from build123d import *

# Parameters (mm, degrees)
SKETCH1_W           = 35
SKETCH1_H           = 35
BOSS_EXTRUDE1_DEPTH = 32
SKETCH2_R           = 16
SKETCH2_R_2         = 10.1
BOSS_EXTRUDE2_DEPTH = 10
SKETCH3_R           = 10
CUT_EXTRUDE1_DEPTH  = 25
SKETCH4_R           = 2
CUT_EXTRUDE2_DEPTH  = 20
SKETCH5_R           = 2
CUT_EXTRUDE3_DEPTH  = 20
SKETCH6_W           = 25
SKETCH6_H           = 25
SKETCH6_W_2         = 20.1
SKETCH6_H_2         = 20.1
BOSS_EXTRUDE3_DEPTH = 25
SKETCH7_R           = 2.5
CUT_EXTRUDE4_DEPTH  = 60.956234102
SKETCH8_R           = 2.5
CUT_EXTRUDE5_DEPTH  = 25
FILLET1_R           = 2
FILLET2_R           = 2
FILLET3_R           = 1
CHAMFER1_SIZE       = 2


with BuildPart() as part:
    # Sketch1 → Boss-Extrude1 (new body)
    with BuildSketch(Plane.XY):
        Rectangle(SKETCH1_W, SKETCH1_H)
    extrude(amount=BOSS_EXTRUDE1_DEPTH)

    # Sketch2 → Boss-Extrude2 (add)
    with BuildSketch(Plane(origin=(0, 0, 0), x_dir=(-1, 0, 0), z_dir=(0, 0, -1))):
        Circle(SKETCH2_R)
        Circle(SKETCH2_R_2, mode=Mode.SUBTRACT)
    extrude(amount=BOSS_EXTRUDE2_DEPTH)

    # Sketch3 → Cut-Extrude1 (cut)
    with BuildSketch(Plane(origin=(0, 0, 0), x_dir=(-1, 0, 0), z_dir=(0, 0, -1))):
        Circle(SKETCH3_R)
    extrude(amount=-CUT_EXTRUDE1_DEPTH, mode=Mode.SUBTRACT)

    # Sketch4 → Cut-Extrude2 (cut, symmetric)
    with BuildSketch(Plane(origin=(0, 0, 0), x_dir=(1, 0, 0), z_dir=(0, 1, 0))):
        with Locations(Location((0, 5, 0), (0, 0, 270))):
            Circle(SKETCH4_R)
    extrude(amount=CUT_EXTRUDE2_DEPTH, both=True, mode=Mode.SUBTRACT)

    # Sketch5 → Cut-Extrude3 (cut, symmetric)
    with BuildSketch(Plane(origin=(0, 0, 0), x_dir=(0, 0, -1), z_dir=(1, 0, 0))):
        with Locations((5, 0)):
            Circle(SKETCH5_R)
    extrude(amount=CUT_EXTRUDE3_DEPTH, both=True, mode=Mode.SUBTRACT)

    # Sketch6 → Boss-Extrude3 (add)
    with BuildSketch(Plane(origin=(0, 17.5, 0), x_dir=(1, 0, 0), z_dir=(0, 1, 0))):
        with Locations((0, -16)):
            Rectangle(SKETCH6_W, SKETCH6_H)
        with Locations((0, -16)):
            Rectangle(SKETCH6_W_2, SKETCH6_H_2, mode=Mode.SUBTRACT)
    extrude(amount=BOSS_EXTRUDE3_DEPTH)

    # Sketch7 → Cut-Extrude4 (cut, through all)
    with BuildSketch(Plane.XY.offset(28.5)):
        with Locations((0, 30)):
            Circle(SKETCH7_R)
    extrude(amount=-CUT_EXTRUDE4_DEPTH, mode=Mode.SUBTRACT)

    # Sketch8 → Cut-Extrude5 (cut)
    with BuildSketch(Plane(origin=(12.5, 0, 0), x_dir=(0, 0, -1), z_dir=(1, 0, 0))):
        with Locations((-16, 30)):
            Circle(SKETCH8_R)
    extrude(amount=-CUT_EXTRUDE5_DEPTH, mode=Mode.SUBTRACT)

    # Fillet1
    fillet1_edges = [part.edges().sort_by_distance(p)[0] for p in [
        (-12.5, 30, 3.5),
        (-12.5, 30, 28.5),
        (12.5, 30, 28.5),
        (12.5, 30, 3.5),
        (-17.5, 17.5, 16),
        (17.5, 17.5, 16),
    ]]
    fillet(fillet1_edges, radius=FILLET1_R)

    # Fillet2
    fillet2_edges = [part.edges().sort_by_distance(p)[0] for p in [
        (17.5, -17.5, 16),
        (-17.5, -17.5, 16),
    ]]
    fillet(fillet2_edges, radius=FILLET2_R)

    # Fillet3
    fillet3_edges = [part.edges().sort_by_distance(p)[0] for p in [
        (16, 0, 0),
    ]]
    fillet(fillet3_edges, radius=FILLET3_R)

    # Chamfer1
    chamfer1_edges = [part.edges().sort_by_distance(p)[0] for p in [
        (-12.5, 17.5, 16),
        (0, 17.5, 3.5),
        (12.5, 17.5, 16),
        (0, 17.5, 28.5),
        (11.914213562, 17.5, 27.914213562),
        (11.914213562, 17.5, 4.085786438),
        (-11.914213562, 17.5, 4.085786438),
        (-11.914213562, 17.5, 27.914213562),
    ]]
    chamfer(chamfer1_edges, length=CHAMFER1_SIZE)


solid = part.part
Verification items for the finished model (mm, model axes). A direction names the side the tool comes from. Coordinates: 2 decimals unless noted, no trailing zeros. Loops run counter-clockwise (first coordinate to the right, second up) from the corner with the lowest first, then second, coordinate; pieces in that order, holes last. Notation, with made-up numbers: (45.25, 14.25) -> (55.25, 14.25) arc R21 cw to (55.25, 29.25) -> close; hole circle Ø1 at (44.5, 74.5). An arc over 180 degrees is marked (long way). Write each question's results on one line, items separated by ' | '.
Item 1: Section check C-C, the plane y = 0. Enter the section's corners in (x, z), plus the area to 3 significant figures.
Found:
outline: (-17.5, 0) -> (-17, 0) arc R1 cw to (-16, -1) -> (-16, -3) -> (-10.1, -3) -> (-10.1, 0) -> (-10, 0) -> (-10, 25) -> (10, 25) -> (10, 0) -> (10.1, 0) -> (10.1, -3) -> (16, -3) -> (16, -1) arc R1 cw to (17, 0) -> (17.5, 0) -> (17.5, 32) -> (-17.5, 32) -> close; (-16, -10) -> (-10.1, -10) -> (-10.1, -7) -> (-16, -7) -> close; (10.1, -10) -> (16, -10) -> (16, -7) -> (10.1, -7) -> close | area: 691 mm2
Item 2: Gauge pin test, flat ends, axial feed: pin 1 (17 mm diameter, centred on y = 33, z = 16, fed in from +X); pin 2 (16 mm diameter, centred on x = 0, y = 0, fed in from -Z); pin 3 (16 mm diameter, centred on x = -0.5, z = 15.5, fed in from +Y); pin 4 (4.5 mm diameter, centred on x = 0, y = 30, fed in from +Z). Record the tip position at first contact, or that the pin passes through.
Found:
pin 1: stops at x = 12.5 | pin 2: stops at z = 25 | pin 3: stops at y = 17.5 | pin 4: passes through
Item 3: Material ranges on L1, parallel to Y at x = 0, z = 5.4; L2, parallel to Z at x = -7.5, y = 20.5; L3, parallel to X at y = 35.5, z = 10.5, recorded low to high.
Found:
L1: y = -17.5 to -10, 10 to 27.5, 32.5 to 42.5 | L2: z = 3.5 to 5.95, 26.05 to 28.5 | L3: x = -12.5 to -10.05, 10.05 to 12.5
Item 4: Mould release check, pull along X, two halves, no side actions. Record for faces 6 (the face through (0, 0, 25)), 7 (the face through (-7.9, -15.5, 0)), 8 (the face through (12.433, 18.736, 3.524)): +X half, -X half, draft (parallel to the pull), parting line (faces both ways), or undercut.
Found:
face 6: undercut | face 7: draft | face 8: +X half
Item 5: Section check B-B, the plane y = 20.5. Enter the section's corners in (x, z), plus the area to 3 significant figures.
Found:
outline: (-12.5, 5.5) arc R2 ccw to (-10.5, 3.5) -> (10.5, 3.5) arc R2 ccw to (12.5, 5.5) -> (12.5, 26.5) arc R2 ccw to (10.5, 28.5) -> (-10.5, 28.5) arc R2 ccw to (-12.5, 26.5) -> close; hole (-10.05, 5.95) -> (10.05, 5.95) -> (10.05, 26.05) -> (-10.05, 26.05) -> close | area: 218 mm2
Item 6: Section check D-D, the plane z = 8. Enter the section's corners in (x, y).
Found:
outline: (-17.5, -15.5) arc R2 ccw to (-15.5, -17.5) -> (15.5, -17.5) arc R2 ccw to (17.5, -15.5) -> (17.5, 15.5) arc R2 ccw to (15.5, 17.5) -> (14.5, 17.5) -> (12.5, 19.5) -> (12.5, 42.5) -> (10.05, 42.5) -> (10.05, 17.5) -> (-10.05, 17.5) -> (-10.05, 42.5) -> (-12.5, 42.5) -> (-12.5, 19.5) -> (-14.5, 17.5) -> (-15.5, 17.5) arc R2 ccw to (-17.5, 15.5) -> close; hole circle Ø20 at (0, 0)
Item 7: Section check A-A, the plane z = 16. Enter the section's corners in (x, y).
Found:
outline: (-17.5, -15.5) arc R2 ccw to (-15.5, -17.5) -> (15.5, -17.5) arc R2 ccw to (17.5, -15.5) -> (17.5, 15.5) arc R2 ccw to (15.5, 17.5) -> (14.5, 17.5) -> (12.5, 19.5) -> (12.5, 27.5) -> (10.05, 27.5) -> (10.05, 17.5) -> (-10.05, 17.5) -> (-10.05, 27.5) -> (-12.5, 27.5) -> (-12.5, 19.5) -> (-14.5, 17.5) -> (-15.5, 17.5) arc R2 ccw to (-17.5, 15.5) -> close; (-12.5, 32.5) -> (-10.05, 32.5) -> (-10.05, 42.5) -> (-12.5, 42.5) -> close; (10.05, 32.5) -> (12.5, 32.5) -> (12.5, 42.5) -> (10.05, 42.5) -> close; hole circle Ø20 at (0, 0)
Item 8: Tool access check on faces 1 (the face through (11.93, 31.16, 4.1)), 2 (the face through (-12.5, 33, 16)), 3 (the face through (-10.05, 27, 16)), 4 (the face through (-4.66, -8.96, -4.93)), 5 (the face through (-11.9, 31.16, 27.93)). Record the directions out of +Z, -Z, +X, -X, +Y, -Y that give a thin tool (end or side, any length) a straight path to the whole face; none if there is none.
Found:
face 1: -Z, +X, +Y | face 2: +Z, -Z, -X, +Y | face 3: +Y | face 4: -Z | face 5: +Z, -X, +Y
